For this review, take the finished solid that the model builds, in its own axes (mm). A direction names the side the tool comes from. Coordinates: 2 decimals unless noted, no trailing zeros. Write each loop counter-clockwise with the first axis right and the second up, starting at its lowest first coordinate (ties: lowest second). Pieces come first, ordered by that corner, then holes. Notation, with made-up numbers: (-5, 8) -> (30, 8) arc R29 ccw to (30, 28) -> close; hole circle Ø11 at (-16.5, 77). An arc over 180 degrees is marked (long way). One line per item, written item: value. Start each with the question number.
1) Add section D-D (y = 2). State the section outline as (x, z) points (3 decimals).
2) Add section C-C (x = 61.95). State the section outline as (y, z) points.
3) For probe 1 along X at (y, z) = (3.85, 0) (3 decimals); probe 2 along Z at (x, y) = (61.95, 2.25); probe 3 along Z at (x, y) = (94, 0.9), list the stretches that pass through material, from the lowest coordinate up. Write a range as from..to.
4) Mouldability with a two-part tool opening along X and no side actions: class faces 4 (the flat face through (129, 3, 1)), 5 (the flat face through (115.805, 2.958, -8.198)), 6 (the flat face through (39, 3, 13)) as released by +X, released by -X, zero draft, split by the parting line, or undercut.
5) For pin 1 Ø1.8 at (x, y) = (110, 4) entering from +Z; pin 2 Ø1.8 at (x, y) = (29.5, 2.5) entering from -Z; pin 3 Ø3 at (x, y) = (125.5, 3.5) entering from -Z; pin 4 Ø3 at (x, z) = (12.35, 0) entering from +Y, all flat-tipped, find the tip position at first contact; note any pin that passes through.
6) Add section B-B (z = 0). State the section outline as (x, y) points (3 decimals), and give its area (3 significant figures).
7) Add section A-A (z = 7). State the section outline as (x, y) points, and give its area (3 significant figures).
8) Machinability: for faces 1 (the flat face through (118, 3, 9)), 2 (the flat face through (38, 3, -13)), 3 (the flat face through (98.628, 2.958, -9.769)), which of the approach directions +Z, -Z, +X, -X, +Y, -Y give a long, thin tool a straight path to every point of the face, cutting with its end or side? Answer none if there is none.
from build123d import *

# Parameters (mm, degrees)
BOSS_EXTRUDE1_DEPTH = 6
SKETCH2_R           = 2.45
SKETCH2_R_2         = 2.375
SKETCH2_R_3         = 2.25
CUT_EXTRUDE1_DEPTH  = 7


with BuildPart() as part:
    # Sketch1 → Boss-Extrude1 (new body)
    with BuildSketch(Plane(origin=(0, 0, 0), x_dir=(1, 0, 0), z_dir=(0, 1, 0))):
        Polygon((10, 13), (67, 13), (74, 20), (95.669872981, 20), (95.669872981, 14.892304845), (101.669872981, 4.5), (113.669872981, 4.5), (118, 12), (129, 12), (129, -14), (118, -14), (118, -4.5), (98, -4.5), (98, -20), (74, -20), (67, -13), (10, -13), (0, -3), (0, 3), align=None)
    extrude(amount=BOSS_EXTRUDE1_DEPTH)

    # Sketch2 → Cut-Extrude1 (cut, through all)
    with BuildSketch(Plane(origin=(0, 6, 0), x_dir=(1, 0, 0), z_dir=(0, 1, 0))):
        with Locations((12.35, 0)):
            Circle(SKETCH2_R)
        with Locations((40.65, 0)):
            Circle(SKETCH2_R_2)
        with Locations((61.95, 0)):
            Circle(SKETCH2_R)
        with Locations((94, 0)):
            Circle(SKETCH2_R_3)
        with Locations((122, 0)):
            Circle(SKETCH2_R_3)
    extrude(amount=-CUT_EXTRUDE1_DEPTH, mode=Mode.SUBTRACT)


solid = part.part
Numbers:
1. outline: (0, -3) -> (10, -13) -> (67, -13) -> (74, -20) -> (95.67, -20) -> (95.67, -14.892) -> (101.67, -4.5) -> (113.67, -4.5) -> (118, -12) -> (129, -12) -> (129, 14) -> (118, 14) -> (118, 4.5) -> (98, 4.5) -> (98, 20) -> (74, 20) -> (67, 13) -> (10, 13) -> (0, 3) -> close; hole circle Ø4.9 at (12.35, 0); hole circle Ø4.75 at (40.65, 0); hole circle Ø4.9 at (61.95, 0); hole circle Ø4.5 at (94, 0); hole circle Ø4.5 at (122, 0)
2. outline: (0, -13) -> (6, -13) -> (6, -2.45) -> (0, -2.45) -> close; (0, 2.45) -> (6, 2.45) -> (6, 13) -> (0, 13) -> close
3. probe 1: 0..9.9, 14.8..38.275, 43.025..59.5, 64.4..91.75, 96.25..119.75, 124.25..129
3. probe 2: -13..-2.45, 2.45..13
3. probe 3: -20..-2.25, 2.25..20
4. face 4: released by +X
4. face 5: undercut
4. face 6: zero draft
5. pin 1: z = 4.5
5. pin 2: z = -13
5. pin 3: z = -12
5. pin 4: through
6. outline: (0, 0) -> (9.9, 0) -> (9.9, 6) -> (0, 6) -> close; (14.8, 0) -> (38.275, 0) -> (38.275, 6) -> (14.8, 6) -> close; (43.025, 0) -> (59.5, 0) -> (59.5, 6) -> (43.025, 6) -> close; (64.4, 0) -> (91.75, 0) -> (91.75, 6) -> (64.4, 6) -> close; (96.25, 0) -> (119.75, 0) -> (119.75, 6) -> (96.25, 6) -> close; (124.25, 0) -> (129, 0) -> (129, 6) -> (124.25, 6) -> close
6. area: 633 mm²
7. outline: (4, 0) -> (98, 0) -> (98, 6) -> (4, 6) -> close; (118, 0) -> (129, 0) -> (129, 6) -> (118, 6) -> close
7. area: 630 mm²
8. face 1: +Z, +Y, -Y
8. face 2: -Z, -X, +Y, -Y
8. face 3: -Z, +Y, -Y
